Autodesk Inventor part; units mm, degrees
ref_plane "YZ Plane" through (0, 0, 0) normal (1, 0, 0) x (0, 1, 0)
ref_plane "XZ Plane" through (0, 0, 0) normal (0, 1, 0) x (-1, 0, 0)
ref_plane "XY Plane" through (0, 0, 0) normal (0, 0, 1) x (1, 0, 0)
sketch "Sketch1" plane through (0, 0, 0) normal (0, 0, 1) x (1, 0, 0)
  line L0 (144, 0) -> (0, 0)
  line L1 (0, 0) -> (0, 24)
  line L2 (0, 24) -> (144, 24)
  line L3 (144, 24) -> (144, 0)
  point P0 (0, 0)
  dimension "d0" = 144
  dimension "d1" = 24
extrude "Extrusion1" add sketch "Sketch1" along normal blind 8
sketch "Sketch5" plane through (0, 0, 8) normal (0, 0, 1) x (1, 0, 0)
  circle A0 centre (136, 20) radius 2.5
  line L0 (144, 20) -> (0, 20) construction
  line L1 (136, 24) -> (136, 0) construction
  line L2 (144, 24) -> (0, 24) construction
  line L3 (0, 0) -> (144, 0) construction
  line L4 (0, 24) -> (144, 24) construction
  line L5 (144, 24) -> (144, 0) construction
  line L6 (144, 0) -> (0, 0) construction
  line L7 (0, 0) -> (0, 24) construction
  circle A1 centre (120, 20) radius 2.5
  circle A2 centre (104, 20) radius 2.5
  circle A3 centre (88, 20) radius 2.5
  circle A4 centre (72, 20) radius 2.5
  circle A5 centre (56, 20) radius 2.5
  circle A6 centre (40, 20) radius 2.5
  circle A7 centre (24, 20) radius 2.5
  circle A8 centre (8, 20) radius 2.5
  circle A9 centre (136, 4) radius 2.5
  circle A10 centre (120, 4) radius 2.5
  circle A11 centre (104, 4) radius 2.5
  circle A12 centre (88, 4) radius 2.5
  circle A13 centre (72, 4) radius 2.5
  circle A14 centre (56, 4) radius 2.5
  circle A15 centre (40, 4) radius 2.5
  circle A16 centre (24, 4) radius 2.5
  circle A17 centre (8, 4) radius 2.5
  dimension "d30" = 5
  dimension "d83" = 4
  dimension "d84" = 8
  dimension "d87" = 16
  dimension "d90" = 16
extrude "Extrusion8" cut sketch "Sketch5" against normal through all
sketch "Sketch9" plane through (144, 0, 0) normal (1, 0, 0) x (0, 0, -1)
  circle A0 centre (-4, 20) radius 2
  circle A1 centre (-4, 4) radius 2
  line L0 (0, 0) -> (-8, 0)
  line L1 (0, 24) -> (-8, 24) construction
  line L2 (-8, 24) -> (0, 24) construction
  line L3 (0, 24) -> (0, 0) construction
  line L4 (0, 0) -> (-8, 0) construction
  line L5 (-8, 0) -> (-8, 24) construction
  point P0 (0, 0)
  dimension "d95" = 4
  dimension "d96" = 4
  dimension "d97" = 4
  dimension "d98" = 4
  dimension "d99" = 4
  dimension "d100" = 4
extrude "Extrusion9" cut sketch "Sketch9" against normal blind 4
sketch "Sketch10" plane through (0, 0, 0) normal (-1, 0, 0) x (0, 0, 1)
  line L0 (0, 24) -> (0, 0) construction
  line L1 (0, 24) -> (8, 24) construction
  line L2 (8, 24) -> (8, 0) construction
  line L3 (8, 0) -> (0, 0) construction
  line L4 (0, 0) -> (0, 24) construction
  circle A0 centre (4, 20) radius 2
  circle A1 centre (4, 4) radius 2
  point P0 (0, 0)
  dimension "d107" = 4
  dimension "d108" = 4
  dimension "d109" = 4
  dimension "d110" = 4
  dimension "d111" = 4
  dimension "d112" = 4
extrude "Extrusion10" cut sketch "Sketch10" against normal blind 4
sketch "Sketch11" plane through (0, 0, 0) normal (0, 0, -1) x (-1, 0, 0)
  line L0 (-144, 24) -> (-144, 0)
  line L1 (-144, 14) -> (0, 14)
  line L2 (0, 14) -> (0, 10)
  line L3 (0, 10) -> (-144, 10)
  line L4 (-144, 10) -> (-144, 14)
  line L5 (0, 24) -> (-144, 24)
  line L6 (-144, 0) -> (0, 0)
  point P0 (0, 0)
  dimension "d119" = 10
  dimension "d120" = 10
  dimension "d121" = 144
extrude "Extrusion11" cut sketch "Sketch11" against normal blind 6
properties part number "Beam0824-144-Blue" material "Aluminum 6061"
The listing builds one solid part. Answer for the finished solid, in the listing's coordinates (mm). A direction names the side the tool comes from. Give positions to 0.01 mm unless a question says otherwise; leave off trailing zeros. Loops run counter-clockwise (first coordinate to the right, second up) from the corner with the lowest first, then second, coordinate; pieces in that order, holes last. Notation, with made-up numbers: (37, 42) - (89, 42) arc R12 ccw to (89, 60) - close; hole circle Ø3 at (-1, 66). An arc over 180 degrees is marked (long way). Answer as a JSON object with one key per item and string values.
1. Find the intervals of material crossed by L1, parallel to Y at x = 120, z = 4.5; L2, parallel to Y at x = 2.5, z = 4; L3, parallel to Y at x = 27.5, z = 2.75, in increasing order. Write a range as [from, to].
Determined:
{"L1": "[0, 1.5], [6.5, 10], [14, 17.5], [22.5, 24]", "L2": "[0, 2], [6, 10], [14, 18], [22, 24]", "L3": "[0, 10], [14, 24]"}
2. A cutting plane is placed at B-B (z = 4). Give the number of separate pieces and of enclosed holes in the cut face, then the cut area to 3 significant figures.
Determined:
{"separate pieces": "2", "enclosed holes": "18", "area": "2,460 mm²"}
3. A cutting plane is placed at A-A (x = 88). Write down the section's boundary in (y, z).
Determined:
{"outline": "(0, 0) - (1.5, 0) - (1.5, 8) - (0, 8) - close; (6.5, 0) - (10, 0) - (10, 6) - (14, 6) - (14, 0) - (17.5, 0) - (17.5, 8) - (6.5, 8) - close; (22.5, 0) - (24, 0) - (24, 8) - (22.5, 8) - close"}
4. Flat-ended cylindrical pins translate along their axes: pin 1 Ø4.5 at (x, y) = (8, 20) entering from -Z; pin 2 Ø3.5 at (y, z) = (4, 4) entering from +X. Find the tip coordinate at first contact, or state that the pin passes through.
Determined:
{"pin 1": "through", "pin 2": "x = 140"}
5. For faces 1 (the cylindrical face through (2, 22, 4)), 2 (the cylindrical face through (142, 2.8, 5.6)), 3 (the flat face through (73, 12, 6)), determine the directions among +Z, -Z, +X, -X, +Y, -Y from which every point of the face is accessible in a straight line to the end or side of a thin tool.
Determined:
{"face 1": "-X", "face 2": "+X", "face 3": "-Z, +X, -X"}
6. For a pull along X with two mould halves and no side action, classify faces 4 (the flat face through (144, 12, 7)), 5 (the cylindrical face through (22.16, 5.69, 4.06)), 6 (the flat face through (71, 17, 0)) as pulls with the +X half, pulls with the -X half, needs draft (parallel to the pull), parting line crosses it, or undercut.
Determined:
{"face 4": "pulls with the +X half", "face 5": "undercut", "face 6": "needs draft"}
7. A cutting plane is placed at D-D (x = 9). Write down the section's boundary in (y, z), then the cut area to 3 significant figures.
Determined:
{"outline": "(0, 0) - (1.71, 0) - (1.71, 8) - (0, 8) - close; (6.29, 0) - (10, 0) - (10, 6) - (14, 6) - (14, 0) - (17.71, 0) - (17.71, 8) - (6.29, 8) - close; (22.29, 0) - (24, 0) - (24, 8) - (22.29, 8) - close", "area": "94.7 mm²"}
